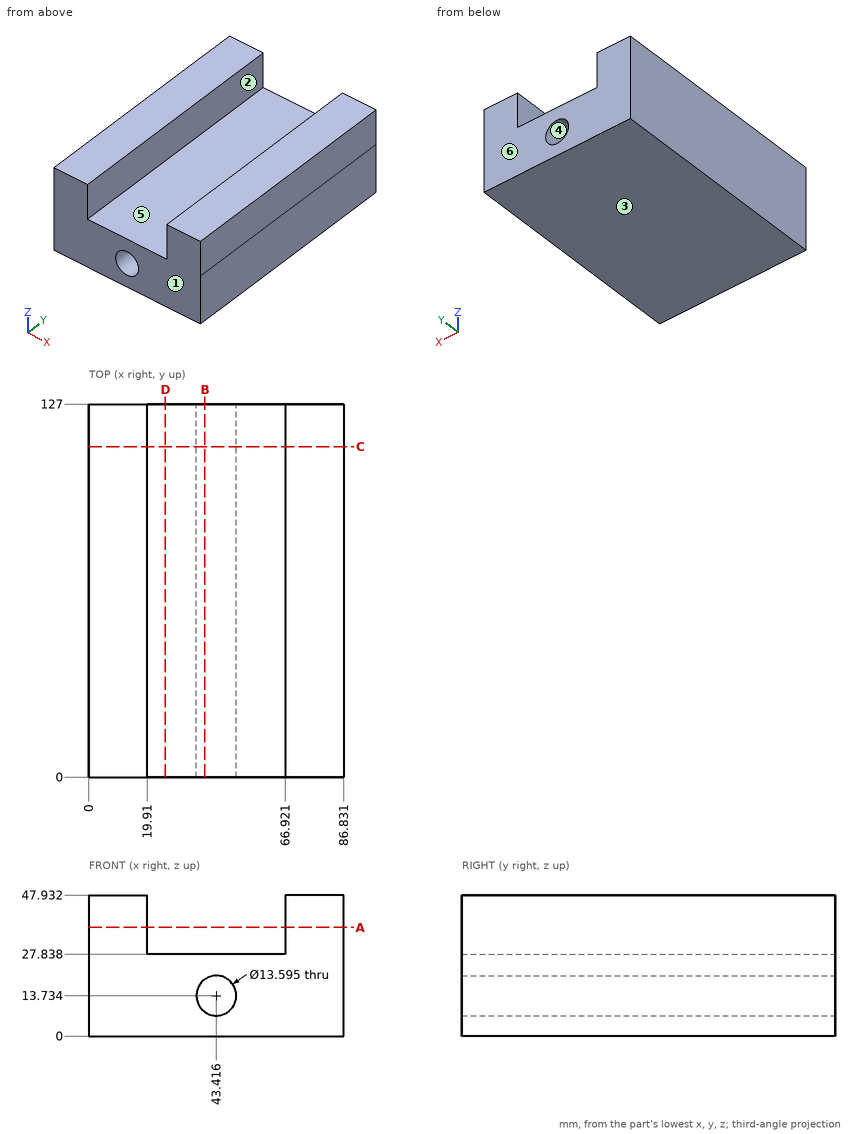
Answer from the drawing. Dimensions are ordinates in mm from the lowest x, y and z of the part. A direction names the side the tool comes from. Round coordinates to 2 decimals unless told otherwise and drop trailing zeros. Write each loop counter-clockwise with the first axis right and the second up, starting at its lowest first coordinate (ties: lowest second). Pieces come first, ordered by that corner, then holes. Notation, with made-up numbers: (54.25, 14) -> (106.25, 14) arc R11 cw to (106.25, 19) -> close; hole circle Ø6 at (82, 30). An arc over 180 degrees is marked (long way). Write each question's results on one line, items separated by ' | '.
1) Flat-ended cylindrical pins translate along their axes: pin 1 (2 mm diameter, centred on x = 48, y = 101.5, fed in from -Z); pin 2 (4 mm diameter, centred on x = 33.5, y = 42, fed in from +Z). Find the tip coordinate at first contact, or state that the pin passes through.
Findings:
pin 1: stops at z = 0 | pin 2: stops at z = 27.84
2) The part is cut by section A-A (z = 37). Write down the section's boundary in (x, y), and give its area (3 significant figures).
Findings:
outline: (0, 0) -> (19.91, 0) -> (19.91, 127) -> (0, 127) -> close; (66.92, 0) -> (86.83, 0) -> (86.83, 127) -> (66.92, 127) -> close | area: 5,060 mm²
3) Which of the six approach directions +Z, -Z, +X, -X, +Y, -Y give full straight-line access (tool end or side, diameter ignored) to the marked faces 1 and 2?
Findings:
face 1: +Z, -Z, +X, -X, -Y | face 2: +Z, +Y, -Y
4) The part is cut by section B-B (x = 39.5). Write down the section's boundary in (y, z).
Findings:
outline: (0, 0) -> (127, 0) -> (127, 8.18) -> (0, 8.18) -> close; (0, 19.29) -> (127, 19.29) -> (127, 27.84) -> (0, 27.84) -> close
5) The part is cut by section C-C (y = 112.5). Write down the section's boundary in (x, z) (1 decimal).
Findings:
outline: (0, 0) -> (86.8, 0) -> (86.8, 27.8) -> (86.8, 47.9) -> (66.9, 47.9) -> (66.9, 27.8) -> (19.9, 27.8) -> (19.9, 47.9) -> (0, 47.9) -> close; hole circle Ø13.6 at (43.4, 13.7)
6) For a pull along Z with two mould halves and no side action, classify the marked faces 3, 4, 5 and 6 as +Z half, -Z half, draft (parallel to the pull), parting line (faces both ways), or undercut.
Findings:
face 3: -Z half | face 4: undercut | face 5: +Z half | face 6: draft
7) Consider line 1 along X through (y, z) = (57.5, 45.5); line 2 along Z through (x, y) = (28.5, 49); line 3 along X through (y, z) = (121.5, 17.5) (1 decimal). Determine where each line is inside the solid, lowest interval first. Write a range as [from, to].
Findings:
line 1: x = [0, 19.91], [66.92, 86.83] | line 2: z = [0, 27.84] | line 3: x = [0, 37.8], [49.1, 86.8]
8) The part is cut by section D-D (x = 26). Write down the section's boundary in (y, z), and give its area (3 significant figures).
Findings:
outline: (0, 0) -> (127, 0) -> (127, 27.84) -> (0, 27.84) -> close | area: 3,540 mm²
